The model under review builds one solid part; all positions refer to its coordinate system, in mm. A direction names the side the tool comes from. Give positions to 0.01 mm unless a question says otherwise; leave off trailing zeros. Loops run counter-clockwise (first coordinate to the right, second up) from the corner with the lowest first, then second, coordinate; pieces in that order, holes last. Notation, with made-up numbers: (73, 48.25) -> (122, 48.25) arc R17 cw to (122, 52.25) -> close; hole circle Ø9 at (36.5, 32.25). An arc over 180 degrees is marked (long way). Write each question's results on one line, items separated by ' | '. Start each with the question number.
Q1. We need section B-B (x = -11.5). Write out the cut boundary in (y, z).
Q2. Insertion check: pin 1 Ø9.5 at (x, y) = (18, 14) entering from +Z; pin 2 Ø10 at (x, z) = (21, -6) entering from +Y; pin 3 Ø1.5 at (y, z) = (20, -5) entering from -X. Each pin has a flat end and moves straight along its axis. Give the tip position at first contact, or say it passes through.
Q3. We need section D-D (x = 16). Write out the cut boundary in (y, z).
Q4. Mouldability with a two-part tool opening along X and no side actions: class faces 1 (the face through (49.229, 26, 3)), 2 (the face through (-23.91, 6.82, -7.22)), 3 (the face through (34, 14.224, 3)) as released by +X, released by -X, zero draft, split by the parting line, or undercut.
Q5. We need section A-A (y = 3). Write out the cut boundary in (x, z) (3 decimals), plus the area to 3 significant figures.
Q6. We need section C-C (y = 19). Write out the cut boundary in (x, z).
Q7. Wall thickness on L1, parallel to Z at x = -16.5, y = 9; L2, parallel to X at y = 11, z = 10; L3, parallel to Y at x = 12, z = 13: over which ranges is each line inside the solid? List them lowest first. Write a range as [from, to].
Q8. Machinability: for faces 4 (the face through (30.052, 10, 3)), 5 (the face through (-31.784, 7.672, 2.048)), 6 (the face through (17, 14, -0.474)), 7 (the face through (12, 6.35, 12)), which of the approach directions +Z, -Z, +X, -X, +Y, -Y give a long, thin tool a straight path to every point of the face, cutting with its end or side? Answer none if there is none.
from build123d import *

# Parameters (mm, degrees)
SKETCH4_W                 = 53.975
SKETCH4_H                 = 31.75
BOSS_EXTRUDE1_DEPTH       = 6.35
SKETCH5_R                 = 15.875
BOSS_EXTRUDE2_DEPTH       = 6.35
CUT_EXTRUDE1_DEPTH        = 45.208170155
CUT_EXTRUDE1_DEPTH_BACK   = 45.208170155
SKETCH6_R                 = 9.525
SKETCH7_W                 = 9.525
SKETCH7_H                 = 25.4
BOSS_EXTRUDE3_DEPTH       = 31.75
BOSS_EXTRUDE4_DEPTH       = 9.525
SKETCH9_R                 = 9.525
BOSS_EXTRUDE5_DEPTH       = 11.176
CUT_EXTRUDE2_DEPTH        = 8.001
BOSS_EXTRUDE11_DEPTH      = 3.175
BOSS_EXTRUDE11_DEPTH_BACK = 3.175
BOSS_EXTRUDE12_START      = -6.35
BOSS_EXTRUDE12_DEPTH      = 6.35
CUT_EXTRUDE3_DEPTH        = 68.007319115
CUT_EXTRUDE3_DEPTH_BACK   = 68.007319115
CUT_EXTRUDE5_REACH        = 87.932
CUT_EXTRUDE5_END_RADIUS   = 9.525
SKETCH21_R                = 1.7272
CIRPATTERN1_COUNT         = 2
CIRPATTERN1_ANGLE         = 90
FILLET3_R                 = 0.762
CUT_EXTRUDE6_DEPTH        = 72.659896883
CUT_EXTRUDE6_DEPTH_BACK   = 72.659896883
SKETCH22_R                = 1.7272


with BuildPart() as part:
    # Sketch4 → Boss-Extrude1 (new body)
    with BuildSketch(Plane(origin=(0, 0, 0), x_dir=(1, 0, 0), z_dir=(0, 1, 0))):
        with BuildLine():
            Line((-15.922424051, 13.173838608), (-15.922424051, -18.576161392))
            ThreePointArc((-15.922424051, -18.576161392), (-31.797424051, -2.701161392), (-15.922424051, 13.173838608))
        make_face()
        with Locations((11.065075949, -2.701161392)):
            Rectangle(SKETCH4_W, SKETCH4_H)
    extrude(amount=BOSS_EXTRUDE1_DEPTH)

    # Sketch5 → Boss-Extrude2 (add)
    with BuildSketch(Plane(origin=(0, 6.35, 0), x_dir=(1, 0, 0), z_dir=(0, 1, 0))):
        with Locations(Location((-15.922424051, -2.701161392, 0), (0, 0, 270))):
            Circle(SKETCH5_R)
    extrude(amount=BOSS_EXTRUDE2_DEPTH)

    # Sketch6 → Cut-Extrude1 (cut, two sides: drawn at the far end of the back side and taken through both)
    with BuildSketch(Plane(origin=(0, 12.7, 0), x_dir=(1, 0, 0), z_dir=(0, 1, 0)).offset(-CUT_EXTRUDE1_DEPTH_BACK)):
        with Locations(Location((-15.922424051, -2.701161392, 0), (0, 0, 270))):
            Circle(SKETCH6_R)
    extrude(amount=CUT_EXTRUDE1_DEPTH + CUT_EXTRUDE1_DEPTH_BACK, mode=Mode.SUBTRACT)

    # Sketch7 → Boss-Extrude3 (add)
    with BuildSketch(Plane.XY.offset(18.576161392)):
        with Locations((33.290075949, 12.7)):
            Rectangle(SKETCH7_W, SKETCH7_H)
    extrude(amount=-BOSS_EXTRUDE3_DEPTH)

    # Sketch8 → Boss-Extrude4 (add)
    with BuildSketch(Plane(origin=(38.052575949, 0, 0), x_dir=(0, 0, -1), z_dir=(1, 0, 0))):
        with BuildLine():
            Line((-18.576161392, 25.4), (13.173838608, 25.4))
            ThreePointArc((13.173838608, 25.4), (-2.701161392, 41.275), (-18.576161392, 25.4))
        make_face()
    extrude(amount=-BOSS_EXTRUDE4_DEPTH)

    # Sketch9 → Boss-Extrude5 (add)
    with BuildSketch(Plane(origin=(38.052575949, 0, 0), x_dir=(0, 0, -1), z_dir=(1, 0, 0))):
        with Locations((-2.701161392, 25.4)):
            Circle(SKETCH9_R)
    extrude(amount=BOSS_EXTRUDE5_DEPTH)

    # Sketch10 → Cut-Extrude2 (cut)
    with BuildSketch(Plane(origin=(38.052575949, 0, 0), x_dir=(0, 0, -1), z_dir=(1, 0, 0))):
        with BuildLine():
            Line((-13.038961392, 14.224), (7.662038608, 14.224))
            ThreePointArc((7.662038608, 14.224), (8.200853975, 14.000815367), (8.424038608, 13.462))
            Line((8.424038608, 13.462), (8.424038608, 7.112))
            ThreePointArc((8.424038608, 7.112), (8.200853975, 6.573184633), (7.662038608, 6.35))
            Line((7.662038608, 6.35), (-13.038961392, 6.35))
            ThreePointArc((-13.038961392, 6.35), (-13.57777676, 6.573184633), (-13.800961392, 7.112))
            Line((-13.800961392, 7.112), (-13.800961392, 13.462))
            ThreePointArc((-13.800961392, 13.462), (-13.57777676, 14.000815367), (-13.038961392, 14.224))
        make_face()
    extrude(amount=-CUT_EXTRUDE2_DEPTH, mode=Mode.SUBTRACT)

    # Sketch12 → Boss-Extrude11 (add, two sides: drawn at the far end of the back side and taken through both)
    with BuildSketch(Plane.XY.offset(2.701161392).offset(-BOSS_EXTRUDE11_DEPTH_BACK)):
        Polygon((28.527575949, 6.35), (28.527575949, 25.8550254), (3.102758151, 11.176), (3.102758151, 6.35), align=None)
    extrude(amount=BOSS_EXTRUDE11_DEPTH + BOSS_EXTRUDE11_DEPTH_BACK)

    # Sketch17 → Boss-Extrude12 (add)
    with BuildSketch(Plane(origin=(0, 12.7, 0), x_dir=(1, 0, 0), z_dir=(0, 1, 0)).offset(BOSS_EXTRUDE12_START)):
        with BuildLine():
            Line((3.102758151, 0.473838608), (-0.368164184, 0.473838608))
            ThreePointArc((-0.368164184, 0.473838608), (-0.047424051, -2.701161392), (-0.368164184, -5.876161392))
            Line((-0.368164184, -5.876161392), (3.102758151, -5.876161392))
            Line((3.102758151, -5.876161392), (3.102758151, 0.473838608))
        make_face()
    extrude(amount=BOSS_EXTRUDE12_DEPTH)

    # Sketch19 → Cut-Extrude3 (cut, two sides: drawn at the far end of the back side and taken through both)
    with BuildSketch(Plane(origin=(0, 0, -0.473838608), x_dir=(-1, 0, 0), z_dir=(0, 0, -1)).offset(-CUT_EXTRUDE3_DEPTH_BACK)):
        with BuildLine():
            Line((0.368164184, 12.7), (-3.102758151, 12.7))
            Line((-3.102758151, 12.7), (-3.102758151, 11.176))
            ThreePointArc((-3.102758151, 11.176), (-1.025931877, 11.160538208), (0.368164184, 12.7))
        make_face()
    extrude(amount=CUT_EXTRUDE3_DEPTH + CUT_EXTRUDE3_DEPTH_BACK, mode=Mode.SUBTRACT)

    # Cut-Extrude5: up to this cylinder (the profile starts outside it)
    cut_extrude5_end = Plane(origin=(-15.922424051, 7.874, 2.701161392), z_dir=(0, 1, 0)) * Cylinder(CUT_EXTRUDE5_END_RADIUS, 195.914, mode=Mode.PRIVATE)
    # Sketch21 → Cut-Extrude5 (cut, up to the surface)
    with BuildSketch(Plane(origin=(-27.147744202, 12.7, 13.926481544), x_dir=(0.7071067811865489, 0, 0.7071067811865462), z_dir=(-0.7071067811865462, 0, 0.7071067811865489)), mode=Mode.PRIVATE) as cut_extrude5_sk1:
        with Locations((0, -4.826)):
            Circle(SKETCH21_R)
    cut_extrude5_tool1 = extrude(cut_extrude5_sk1.sketch, amount=-CUT_EXTRUDE5_REACH, mode=Mode.PRIVATE) - cut_extrude5_end
    cut_extrude5 = cut_extrude5_tool1.solids().sort_by_distance((-27.147744, 7.874, 13.926482))[0]
    add(cut_extrude5, mode=Mode.SUBTRACT)

    # CirPattern1: Cut-Extrude5 ×2 about axis
    cirpattern1_axis = Axis((-15.922424051, 0, 2.701161392), (0, -1, 0))
    for i in range(1, CIRPATTERN1_COUNT):
        add(cut_extrude5.rotate(cirpattern1_axis, i * CIRPATTERN1_ANGLE / (CIRPATTERN1_COUNT - 1)), mode=Mode.SUBTRACT)

    # Fillet3
    fillet3_edges = [part.edges().sort_by_distance(p)[0] for p in [
        (28.527575949, 16.1025127, -0.473838608),
        (28.527575949, 16.1025127, 5.876161392),
    ]]
    fillet(fillet3_edges, radius=FILLET3_R)

    # Sketch22 → Cut-Extrude6 (cut, two sides: drawn at the far end of the back side and taken through both)
    with BuildSketch(Plane.XY.offset(18.576161392).offset(-CUT_EXTRUDE6_DEPTH_BACK)):
        with Locations(Location((34.877575949, 10.287, 0), (0, 0, 270))):
            Circle(SKETCH22_R)
    extrude(amount=CUT_EXTRUDE6_DEPTH + CUT_EXTRUDE6_DEPTH_BACK, mode=Mode.SUBTRACT)


solid = part.part
Output:
1) outline: (0, -13.17) -> (6.35, -13.17) -> (6.35, -12.55) -> (12.7, -12.55) -> (12.7, -5.73) -> (0, -5.73) -> close; (0, 11.14) -> (12.7, 11.14) -> (12.7, 17.95) -> (6.35, 17.95) -> (6.35, 18.58) -> (0, 18.58) -> close
2) pin 1: z = 5.88 | pin 2: y = 6.35 | pin 3: x = 28.53
3) outline: (0, -13.17) -> (6.35, -13.17) -> (6.35, -0.47) -> (18.62, -0.47) -> (18.62, 5.88) -> (6.35, 5.88) -> (6.35, 18.58) -> (0, 18.58) -> close
4) face 1: released by +X | face 2: undercut | face 3: zero draft
5) outline: (-15.922, -13.174) -> (38.053, -13.174) -> (38.053, 18.576) -> (-15.922, 18.576) arc R15.875 ccw to start; hole circle Ø19.05 at (-15.922, 2.701) | area: 1,820 mm2
6) outline: (16.65, -0.47) -> (27.77, -0.47) arc R0.76 cw to (28.53, -1.24) -> (28.53, -13.17) -> (38.05, -13.17) -> (38.05, -4.35) -> (49.23, -4.35) -> (49.23, 9.76) -> (38.05, 9.76) -> (38.05, 18.58) -> (28.53, 18.58) -> (28.53, 6.64) arc R0.76 cw to (27.77, 5.88) -> (16.65, 5.88) -> close
7) L1: [-13.16, -6.81], [12.21, 18.57] | L2: [-30.02, -22.04], [-9.8, -1.82], [28.53, 30.05] | L3: [0, 6.35]
8) face 4: +X | face 5: +Y | face 6: -Z, +Y | face 7: +Z, +Y
